```python
from build123d import *

# Parameters (mm, degrees)
EXTRUDE_THIN1_DEPTH = 6
SKETCH3_W           = 327.571594818
SKETCH3_H           = 11.174496413
CUT_EXTRUDE3_DEPTH  = 498.380052114


with BuildPart() as part:
    # Sketch2 → Extrude-Thin1 (new body)
    with BuildSketch(Plane.XY):
        with BuildLine():
            Line((-327.571523016, 7.498350769), (-0.016837352, -0.67478997))
            ThreePointArc((-0.016837352, -0.67478997), (0.476106699, -0.478484494), (0.674865476, 0.013475489))
            Line((0.674865476, 0.013475489), (-0.760216383, 71.883759331))
            ThreePointArc((-0.760216383, 71.883759331), (11.983695064, 85.015150307), (24.987217703, 72.140791802))
            Line((24.987217703, 72.140791802), (24.987217703, -344.844919852))
            ThreePointArc((24.987217703, -344.844919852), (21.212571133, -353.952564578), (12.101906255, -357.719915723))
            Line((12.101906255, -357.719915723), (-332.660093745, -357.443799484))
            ThreePointArc((-332.660093745, -357.443799484), (-341.911283403, -353.512528914), (-345.517294817, -344.129774518))
            Line((-345.517294817, -344.129774518), (-333.717699052, 1.704813786))
            ThreePointArc((-333.717699052, 1.704813786), (-331.836728158, 5.866260785), (-327.571523016, 7.498350769))
        make_face()
        with BuildLine():
            Line((-327.646355689, 4.499284236), (-0.091670025, -3.673856503))
            ThreePointArc((-0.091670025, -3.673856503), (2.592136472, -2.605082247), (3.674267594, 0.07336655))
            Line((3.674267594, 0.07336655), (2.239185734, 71.943650392))
            ThreePointArc((2.239185734, 71.943650392), (12.013642086, 82.015299782), (21.987217703, 72.140791802))
            Line((21.987217703, 72.140791802), (21.987217703, -344.844919852))
            ThreePointArc((21.987217703, -344.844919852), (19.092100431, -351.830394933), (12.104308922, -354.719916685))
            Line((12.104308922, -354.719916685), (-332.657691078, -354.443800446))
            ThreePointArc((-332.657691078, -354.443800446), (-339.753263728, -351.428554087), (-342.519039473, -344.23207256))
            Line((-342.519039473, -344.23207256), (-330.719443707, 1.602515744))
            ThreePointArc((-330.719443707, 1.602515744), (-329.778958261, 3.683239244), (-327.646355689, 4.499284236))
        make_face(mode=Mode.SUBTRACT)
    extrude(amount=EXTRUDE_THIN1_DEPTH)

    # Sketch3 → Cut-Extrude3 (cut, through all)
    with BuildSketch(Plane.XY):
        with Locations((-163.785725607, 1.911102563)):
            Rectangle(SKETCH3_W, SKETCH3_H)
    extrude(amount=CUT_EXTRUDE3_DEPTH, mode=Mode.SUBTRACT)


solid = part.part
```
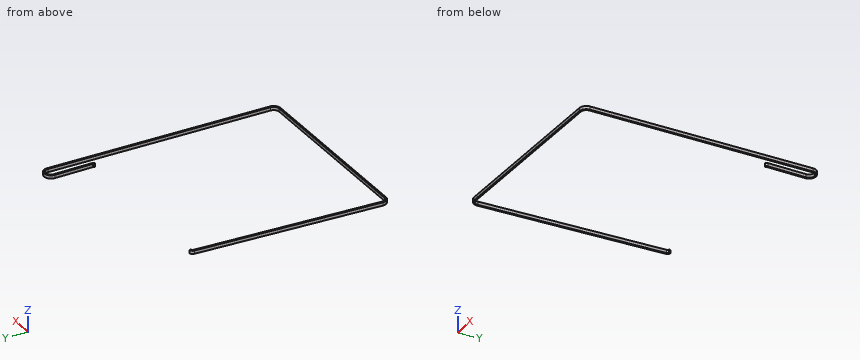
Work out the finished part from the listing and answer in its coordinate system (mm). Round coordinates to 2 decimals unless told otherwise and drop trailing zeros. Loops run counter-clockwise (first coordinate to the right, second up) from the corner with the lowest first, then second, coordinate; pieces in that order, holes last.
(1) The part is cut by section B-B, the plane y = -173.5. Give the vertices of the cut face in (x, z), and give its area (3 significant figures).
Computed values:
outline: (-339.7, 0) - (-336.69, 0) - (-336.69, 6) - (-339.7, 6) - close; (21.99, 0) - (24.99, 0) - (24.99, 6) - (21.99, 6) - close
area: 36.0 mm2
(2) Each of these flat-tipped pins is pushed along its axis until it touches: P1, Ø2, axis at x = -165.5, z = 3.5, coming from the -Y side; P2, Ø1.5, axis at x = -44.5, z = 2.5, coming from the +Y side; P3, Ø0.9, axis at y = -2, z = 4, coming from the -X side. Where does it stop, or does it pass through?
Computed values:
P1: stops at y = -357.58
P2: stops at y = -354.67
P3: stops at x = -333.86
(3) The part is cut by section C-C, the plane x = -303. Give the vertices of the cut face in (y, z).
Computed values:
outline: (-357.47, 0) - (-354.47, 0) - (-354.47, 6) - (-357.47, 6) - close
(4) The part is cut by section A-A, the plane z = 1.95. Give the vertices of the cut face in (x, y) (3 decimals), and give its area (3 significant figures).
Computed values:
outline: (-345.517, -344.13) arc R12.875 ccw to (-332.66, -357.444) - (12.102, -357.72) arc R12.875 ccw to (24.987, -344.845) - (24.987, 72.141) arc R12.875 ccw (long way) to (-0.76, 71.884) - (0.675, 0.013) arc R0.675 cw to (0, -0.675) - (0, -3.675) arc R3.675 ccw to (3.674, 0.073) - (2.239, 71.944) arc R9.875 cw (long way) to (21.987, 72.141) - (21.987, -344.845) arc R9.875 cw to (12.104, -354.72) - (-332.658, -354.444) arc R9.875 cw to (-342.519, -344.232) - (-330.719, 1.603) arc R3 cw to (-327.646, 4.499) - (-327.572, 4.497) - (-327.572, 7.498) arc R6 ccw to (-333.718, 1.705) - close
area: 3,790 mm2
(5) Find the intervals of material crossed by L1, parallel to Y at x = -265.5, z = 0.3; L2, parallel to Y at x = -93, z = 5.05; L3, parallel to X at y = -226.5, z = 1.4, in increasing order.
Computed values:
L1: y = -357.5 to -354.5
L2: y = -357.64 to -354.64
L3: x = -341.5 to -338.5, 21.99 to 24.99
